```python
from build123d import *

# Parameters (mm, degrees)
F0_R     = 10
F0_R_2   = 20
F1_DEPTH = 25.4


with BuildPart() as f1:
    # F0 (on Front) → F1 (new body)
    with BuildSketch(Plane.XZ):
        with BuildLine():
            Line((-43.143227, 76.914711), (-93.143227, 76.914711))
            Line((-93.143227, 76.914711), (-93.143227, 11.914711))
            Line((-93.143227, 11.914711), (-93.143227, -6.085289))
            Line((-93.143227, -6.085289), (-64.090909, -6.085289))
            Line((-64.090909, -6.085289), (-32.130199, -6.085289))
            ThreePointArc((-32.130199, -6.085289), (-21.509733, -10.492569), (-17.13025, -21.124528))
            Line((-17.13025, -21.124528), (-17.143227, -26.085289))
            Line((-17.143227, -26.085289), (6.856773, -26.085289))
            Line((6.856773, -26.085289), (30.856773, -26.085289))
            Line((30.856773, -26.085289), (30.856773, 6.914711))
            Line((30.856773, 6.914711), (30.856773, 46.914711))
            Line((30.856773, 46.914711), (30.856773, 62.914711))
            Line((30.856773, 62.914711), (30.856773, 76.914711))
            Line((30.856773, 76.914711), (25.856773, 76.914711))
            Line((25.856773, 76.914711), (-43.143227, 76.914711))
        make_face()
        with Locations((-63.143227, 11.914711)):
            Circle(F0_R, mode=Mode.SUBTRACT)
        with Locations((6.856773, 6.914711)):
            Circle(F0_R_2, mode=Mode.SUBTRACT)
        with BuildLine():
            ThreePointArc((25.856773, 54.914711), (23.513628, 49.257857), (17.856773, 46.914711))
            Line((17.856773, 46.914711), (-35.143227, 46.914711))
            ThreePointArc((-35.143227, 46.914711), (-40.800081, 49.257857), (-43.143227, 54.914711))
            ThreePointArc((-43.143227, 54.914711), (-40.800081, 60.571565), (-35.143227, 62.914711))
            Line((-35.143227, 62.914711), (17.856773, 62.914711))
            ThreePointArc((17.856773, 62.914711), (23.513628, 60.571565), (25.856773, 54.914711))
        make_face(mode=Mode.SUBTRACT)
    extrude(amount=F1_DEPTH)


solid = f1.part
```
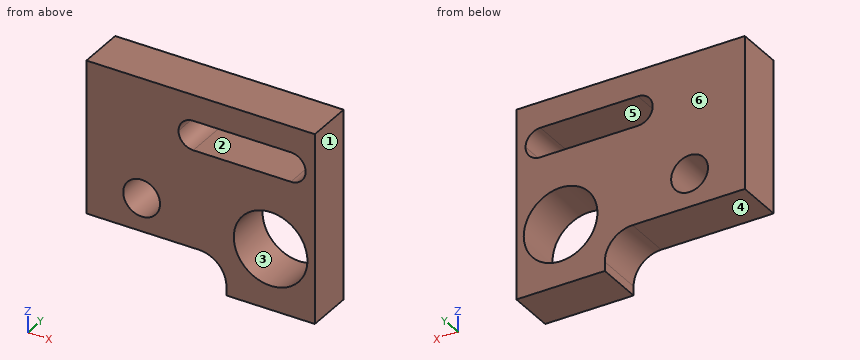
The listing builds one solid part. Answer for the finished solid, in the listing's coordinates (mm). Face numbers are marked on the shaded views. A direction names the side the tool comes from. Give positions to 0.01 mm unless a question says otherwise; leave off trailing zeros. Order: outer loops, then holes, each group sorted by start corner. A loop starts at its lowest first (then second) coordinate and runs counter-clockwise, first axis right, second up. Notation, with made-up numbers: M 56,57.25 L 101,57.25 A25 cw 101,88.25 Z; hole C 0,-18.5 d9. An arc over 180 degrees is marked long. Put each result on its own line as item: value. Start each with the question number.
Item 1: The part is cut by section B-B, the plane z = 25.5. Determine the outline of the cut face in (x, y).
Item 2: Which of the six approach directions +Z, -Z, +X, -X, +Y, -Y give full straight-line access (tool end or side, diameter ignored) to the marked faces 1 and 2?
Item 3: For a pull along Z with two mould halves and no side action, classify the marked faces 3, 4, 5 and 6 as +Z half, -Z half, draft (parallel to the pull), parting line (faces both ways), or undercut.
Item 4: The part is cut by section A-A, the plane x = -9. Determine the outline of the cut face in (y, z), and give its area (3 significant figures).
Item 5: A flat-ended cylindrical pin translates along its axis: P1, Ø4, axis at x = -60.5, z = 36.5, coming from the +Y side. Find the tip coordinate at first contact, or state that the pin passes through.
Item 6: The part is cut by section C-C, the plane x = -55. Determine the outline of the cut face in (y, z).
Item 7: The part is cut by section D-D, the plane y = -16.75. Determine the outline of the cut face in (x, z).
Item 8: Find the intervals of material crossed by line 1 along Z through (x, y) = (-63, -21.5); line 2 along Z through (x, y) = (19.5, -11.5); line 3 along Z through (x, y) = (24.5, -3.75), in increasing order.
Answer key:
1. outline: M -93.14,-25.4 L -0.53,-25.4 L -0.53,0 L -93.14,0 Z; M 14.25,-25.4 L 30.86,-25.4 L 30.86,0 L 14.25,0 Z
2. face 1: +Z, -Z, +X, +Y, -Y
2. face 2: +Y, -Y
3. face 3: undercut
3. face 4: -Z half
3. face 5: undercut
3. face 6: draft
4. outline: M -25.4,-26.09 L 0,-26.09 L 0,-5.27 L -25.4,-5.27 Z; M -25.4,19.1 L 0,19.1 L 0,46.91 L -25.4,46.91 Z; M -25.4,62.91 L 0,62.91 L 0,76.91 L -25.4,76.91 Z
4. area: 1,590 mm²
5. P1: stops at y = 0
6. outline: M -25.4,-6.09 L 0,-6.09 L 0,6.11 L -25.4,6.11 Z; M -25.4,17.72 L 0,17.72 L 0,76.91 L -25.4,76.91 Z
7. outline: M -93.14,-6.09 L -32.13,-6.09 A15 cw -17.13,-21.12 L -17.14,-26.09 L 30.86,-26.09 L 30.86,76.91 L -93.14,76.91 Z; hole C -63.14,11.91 d20; hole M -43.14,54.91 A8 ccw -35.14,46.91 L 17.86,46.91 A8 ccw 25.86,54.91 A8 ccw 17.86,62.91 L -35.14,62.91 A8 ccw Z; hole C 6.86,6.91 d40
8. line 1: z = -6.09 to 1.92, 21.91 to 76.91
8. line 2: z = -26.09 to -8.58, 22.41 to 47.09, 62.74 to 76.91
8. line 3: z = -26.09 to -2.5, 16.33 to 50.46, 59.37 to 76.91
